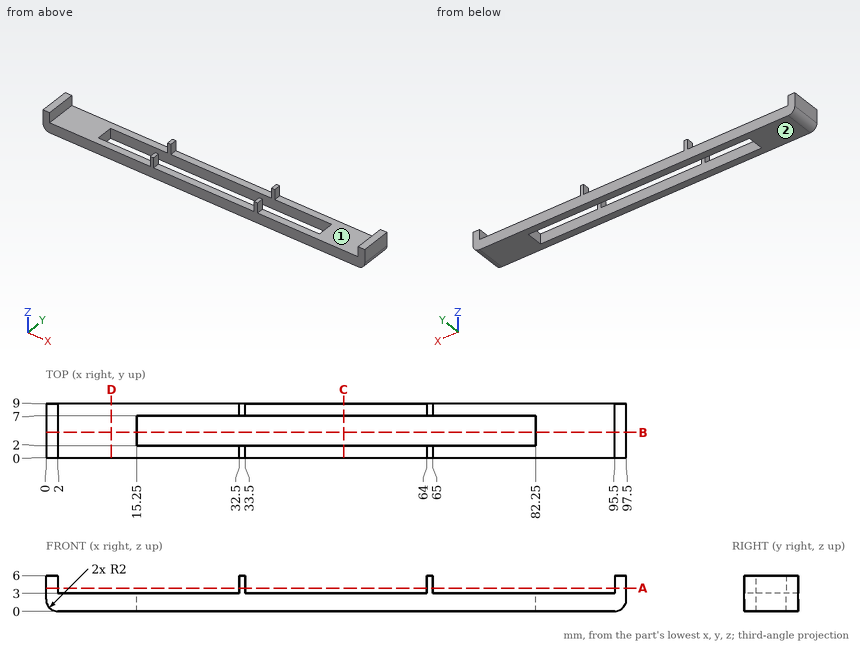
The figure shows three views and two pictorial views of one solid part (mm, origin at its lowest corner). Answer the questions. Coordinates: 2 decimals unless noted, no trailing zeros. Loops run counter-clockwise (first coordinate to the right, second up) from the corner with the lowest first, then second, coordinate; pieces in that order, holes last.
1) Find section B-B on y = 4.25. Write down the section's boundary in (x, z), then the cut area to 3 significant figures.
2) Flat-ended cylindrical pins translate along their axes: pin 1 Ø2 at (x, y) = (55, 1) entering from +Z; pin 2 Ø2 at (x, z) = (12.5, 5) entering from -Y; pin 3 Ø1.5 at (y, z) = (3.5, 1) entering from +X. Find the tip coordinate at first contact, or state that the pin passes through.
3) Determine the mould class of the marked faces 1 and 2 for opening direction X: pulls with the +X half, pulls with the -X half, needs draft (parallel to the pull), parting line crosses it, or undercut.
4) Find section A-A on z = 3.9. Write down the section's boundary in (x, y), then the cut area to 3 significant figures.
5) Find section D-D on x = 11. Write down the section's boundary in (y, z).
6) Find section C-C on x = 50. Write down the section's boundary in (y, z), then the cut area to 3 significant figures.
7) Find the intervals of material crossed by L1, parallel to X at y = 1.5, z = 4; L2, parallel to Y at x = 34.5, z = 1.2; L3, parallel to X at y = 3, z = 5.45, in increasing order.
Values:
1. outline: (0, 2) arc R2 ccw to (2, 0) - (15.25, 0) - (15.25, 3) - (2, 3) - (2, 6) - (0, 6) - close; (82.25, 0) - (95.5, 0) arc R2 ccw to (97.5, 2) - (97.5, 6) - (95.5, 6) - (95.5, 3) - (82.25, 3) - close
1. area: 102 mm2
2. pin 1: stops at z = 3
2. pin 2: passes through
2. pin 3: stops at x = 97.48
3. face 1: undercut
3. face 2: needs draft
4. outline: (0, 0) - (2, 0) - (2, 9) - (0, 9) - close; (32.5, 0) - (33.5, 0) - (33.5, 2) - (32.5, 2) - close; (32.5, 7) - (33.5, 7) - (33.5, 9) - (32.5, 9) - close; (64, 0) - (65, 0) - (65, 2) - (64, 2) - close; (64, 7) - (65, 7) - (65, 9) - (64, 9) - close; (95.5, 0) - (97.5, 0) - (97.5, 9) - (95.5, 9) - close
4. area: 44.0 mm2
5. outline: (0, 0) - (9, 0) - (9, 3) - (0, 3) - close
6. outline: (0, 0) - (2, 0) - (2, 3) - (0, 3) - close; (7, 0) - (9, 0) - (9, 3) - (7, 3) - close
6. area: 12.0 mm2
7. L1: x = 0 to 2, 32.5 to 33.5, 64 to 65, 95.5 to 97.5
7. L2: y = 0 to 2, 7 to 9
7. L3: x = 0 to 2, 95.5 to 97.5
